Design review of the part built by this model. Coordinates are the model's own, in mm. A direction names the side the tool comes from. Coordinates: 2 decimals unless noted, no trailing zeros. Return JSON: item names as keys, results as strings. Group by question number.
```python
from build123d import *

# Parameters (mm, degrees)
BOSS_EXTRUDE1_DEPTH = 5
SKETCH5_W           = 39.175778664
SKETCH5_H           = 11.134274613
CUT_REVOLVE3_ANGLE  = 30
CUT_EXTRUDE2_DEPTH  = 50


with BuildPart() as part:
    # Sketch2 → Boss-Extrude1 (new body)
    with BuildSketch(Plane(origin=(0, 0, 0), x_dir=(1, 0, 0), z_dir=(0, 1, 0))):
        with BuildLine():
            Line((-19.587889332, 4.75), (-19.587889332, 12.891151468))
            Line((-19.587889332, 12.891151468), (19.587889332, 12.891151468))
            Line((19.587889332, 12.891151468), (19.587889332, 4.75))
            Line((19.587889332, 4.75), (18.770336665, -1.514246746))
            ThreePointArc((18.770336665, -1.514246746), (18.737154352, -1.576452374), (18.671177592, -1.601305403))
            Line((18.671177592, -1.601305403), (-18.671177592, -1.601305403))
            ThreePointArc((-18.671177592, -1.601305403), (-18.737154352, -1.576452374), (-18.770336665, -1.514246746))
            Line((-18.770336665, -1.514246746), (-19.587889332, 4.75))
        make_face()
        with BuildLine():
            Line((18.41371442, 0), (18.5, 0))
            ThreePointArc((18.5, 0), (18.535355339, 0.014644661), (18.55, 0.05))
            Line((18.55, 0.05), (18.55, 4.15))
            ThreePointArc((18.55, 4.15), (18.506066017, 4.256066017), (18.4, 4.3))
            Line((18.4, 4.3), (12.307916791, 4.3))
            add(Edge.make_bspline(
                [(12.307916791, 4.3), (9.637425056, 1.440271055), (11.338639539, -1.2)],
                knots=[0, 0, 0, 1, 1, 1], degree=2))
            Line((11.338639539, -1.2), (18.26371442, -1.2))
            ThreePointArc((18.26371442, -1.2), (18.334425098, -1.170710678), (18.36371442, -1.1))
            Line((18.36371442, -1.1), (18.36371442, -0.05))
            ThreePointArc((18.36371442, -0.05), (18.378359081, -0.014644661), (18.41371442, 0))
        make_face(mode=Mode.SUBTRACT)
        with BuildLine():
            Line((-2, 4.3), (-8.307916791, 4.3))
            add(Edge.make_bspline(
                [(-8.307916791, 4.3), (-10.978408526, 1.440271055), (-9.277194043, -1.2)],
                knots=[0, 0, 0, 1, 1, 1], degree=2))
            Line((-9.277194043, -1.2), (-0.75, -1.2))
            add(Edge.make_bspline(
                [(-2, 4.3), (0.166282415, 1.650512873), (-0.75, -1.2)],
                knots=[0, 0, 0, 1, 1, 1], degree=2))
        make_face(mode=Mode.SUBTRACT)
        with BuildLine():
            Line((9.277194043, -1.2), (0.75, -1.2))
            add(Edge.make_bspline(
                [(2, 4.3), (-0.166282415, 1.650512873), (0.75, -1.2)],
                knots=[0, 0, 0, 1, 1, 1], degree=2))
            Line((2, 4.3), (8.307916791, 4.3))
            add(Edge.make_bspline(
                [(8.307916791, 4.3), (10.978408526, 1.440271055), (9.277194043, -1.2)],
                knots=[0, 0, 0, 1, 1, 1], degree=2))
        make_face(mode=Mode.SUBTRACT)
        with BuildLine():
            Line((-12.307916791, 4.3), (-18.4, 4.3))
            ThreePointArc((-18.4, 4.3), (-18.506066017, 4.256066017), (-18.55, 4.15))
            Line((-18.55, 4.15), (-18.55, 0.05))
            ThreePointArc((-18.55, 0.05), (-18.535355339, 0.014644661), (-18.5, 0))
            Line((-18.5, 0), (-18.41371442, 0))
            ThreePointArc((-18.41371442, 0), (-18.378359081, -0.014644661), (-18.36371442, -0.05))
            Line((-18.36371442, -0.05), (-18.36371442, -1.1))
            ThreePointArc((-18.36371442, -1.1), (-18.334425098, -1.170710678), (-18.26371442, -1.2))
            Line((-18.26371442, -1.2), (-11.338639539, -1.2))
            add(Edge.make_bspline(
                [(-12.307916791, 4.3), (-9.637425056, 1.440271055), (-11.338639539, -1.2)],
                knots=[0, 0, 0, 1, 1, 1], degree=2))
        make_face(mode=Mode.SUBTRACT)
    extrude(amount=BOSS_EXTRUDE1_DEPTH)

    # Sketch5 → Cut-Revolve3 (revolve, cut)
    with BuildSketch(Plane(origin=(0, 5, 0), x_dir=(1, 0, 0), z_dir=(0, 1, 0))):
        with Locations((0, -0.817137307)):
            Rectangle(SKETCH5_W, SKETCH5_H)
    revolve(axis=Axis((-19.587889332, 5, -4.75), (1, 0, 0)), revolution_arc=CUT_REVOLVE3_ANGLE, mode=Mode.SUBTRACT)

    # Sketch8 → Cut-Extrude2 (cut)
    with BuildSketch(Plane.ZY.offset(19.587889332)):
        Polygon((4.230476996, 7.111214782), (-14.213063749, 7.925673134), (-16.866621606, -3.135196744), (3.547382894, -3.844563695), align=None)
        with BuildLine():
            Line((-12.891151468, 0), (-12.891151468, 0.4))
            Line((-12.891151468, 0.4), (-12.891151468, 4.6))
            Line((-12.891151468, 4.6), (-12.891151468, 5))
            Line((-12.891151468, 5), (-12.491151468, 5))
            Line((-12.491151468, 5), (-4.75, 5))
            Line((-4.75, 5), (-4.75, 4.203963132))
            add(Edge.make_bspline(
                [(-4.75, 4.203963132), (-2.254573222, 3.559264678), (-0.743625983, 2.686918883), (0.627090158, 1.89553555), (1.401305403, 1.448542169)],
                knots=[0.350361042, 0.350361042, 0.350361042, 0.350361042, 0.350361042, 1, 1, 1, 1, 1], degree=4))
            ThreePointArc((1.401305403, 1.448542169), (1.547715565, 1.302132008), (1.601305403, 1.102132008))
            Line((1.601305403, 1.102132008), (1.601305403, 0.4))
            ThreePointArc((1.601305403, 0.4), (1.484148116, 0.117157288), (1.201305403, 0))
            Line((1.201305403, 0), (-4.75, 0))
            Line((-4.75, 0), (-12.491151468, 0))
            Line((-12.491151468, 0), (-12.891151468, 0))
        make_face(mode=Mode.SUBTRACT)
        with BuildLine():
            Line((-4.75, 5), (-12.491151468, 5))
            add(Edge.make_bspline(
                [(-12.491151468, 5), (-9.778953574, 5), (-7.727997949, 4.833142186), (-6.095824962, 4.551659678), (-4.75, 4.203963132)],
                knots=[0, 0, 0, 0, 0, 0.350361042, 0.350361042, 0.350361042, 0.350361042, 0.350361042], degree=4))
            Line((-4.75, 4.203963132), (-4.75, 5))
        make_face()
    extrude(amount=-CUT_EXTRUDE2_DEPTH, mode=Mode.SUBTRACT)


solid = part.part
```
Item 1: For line 1 (Z direction, x = 17, y = 0.35); line 2 (X direction, y = 2.35, z = -1); line 3 (X direction, y = 2.85, z = -3.25), list the stretches that pass through material, from the lowest coordinate up.
Item 2: For pin 1 (8 mm diameter, centred on x = 13, z = -4.5, fed in from +Y); pin 2 (2 mm diameter, centred on y = 1.5, z = -2, fed in from -X); pin 3 (1 mm diameter, centred on y = 2.5, z = -2, fed in from -X), all flat-tipped, find the tip position at first contact; note any pin that passes through.
Item 3: The part is to be moulded in two halves that separate along Z. For faces 1 (the flat face through (15, 2, -4.3)), 2 (the flat face through (-19.588, 2, -9)), 3 (the flat face through (19.276, 1.605, -2.358)), 4 (the flat face through (0, 2, -12.891)), say which applies: pulls with the +Z half, pulls with the -Z half, needs draft (parallel to the pull), parting line crosses it, or undercut.
Item 4: Add section A-A (z = -1.25). Count the separate pieces of the cut face and the enclosed holes in it, plus the area to 3 significant figures.
Item 5: Machinability: for faces 5 (the flat face through (18.55, 2, -2)), 6 (the flat face through (19.588, 2, -9)), which of the approach directions +Z, -Z, +X, -X, +Y, -Y give a long, thin tool a straight path to every point of the face, cutting with its end or side? Answer none if there is none.
Geometry check:
{
 "1": {"line 1": "-12.89 to -4.3, 1.2 to 1.6", "line 2": "-19.1 to -18.55, -10.68 to -9.94, -0.5 to 0.5, 9.94 to 10.68, 18.55 to 19.1", "line 3": "-19.39 to -18.55, -11.47 to -9.15, -1.27 to 1.27, 9.15 to 11.47, 18.55 to 19.39"},
 "2": {"pin 1": "y = 4.83", "pin 2": "x = -19.36", "pin 3": "x = -19.29"},
 "3": {"face 1": "undercut", "face 2": "needs draft", "face 3": "pulls with the +Z half", "face 4": "pulls with the -Z half"},
 "4": {"separate pieces": "5", "enclosed holes": "0", "area": "11.0 mm^2"},
 "5": {"face 5": "+Y, -Y", "face 6": "+Z, -Z, +X, +Y, -Y"}
}
